Check sheet for the modelled part. Datum: model origin and axes. Units: mm. A direction names the side the tool comes from. Give positions to 0.01 mm unless a question says otherwise; leave off trailing zeros. Write each loop counter-clockwise with the first axis right and the second up, starting at its lowest first coordinate (ties: lowest second). Pieces come first, ordered by that corner, then holes. Notation, with made-up numbers: M -24.5,12.5 L 9.5,12.5 A25 cw 9.5,28.5 Z; hole C 36.5,-31 d2. An arc over 180 degrees is marked long. One line per item, written item: value. Start each with the question number.
from build123d import *

# Parameters (mm, degrees)
CSK_FOR_M3_SFHCS1_AT_2_COUNT = 2
CSK_FOR_M3_SFHCS1_AT_2_PITCH = 17.67766953
CSK_FOR_M3_SFHCS1_AT_3_COUNT = 2
CSK_FOR_M3_SFHCS1_AT_3_PITCH = 25
CSK_FOR_M3_SFHCS1_AT_4_COUNT = 2
CSK_FOR_M3_SFHCS1_AT_4_PITCH = 17.67766953
BOSS_EXTRUDE3_DEPTH          = 10.75
BOSS_EXTRUDE7_DEPTH          = 2
FILLET6_R                    = 5
SKETCH14_R                   = 1.25
CUT_EXTRUDE2_DEPTH           = 13.75
BOSS_EXTRUDE8_DEPTH          = 12.75
SKETCH16_R                   = 1.25
CUT_EXTRUDE3_DEPTH           = 13.75
FILLET8_R                    = 5
SKETCH17_R                   = 1.5
BOSS_EXTRUDE9_DEPTH          = 1.5
SKETCH20_R                   = 11.625
CUT_EXTRUDE4_DEPTH           = 1.5


with BuildPart() as part:
    # Sketch1 → Revolve1 (revolve)
    with BuildSketch(Plane(origin=(0, 0, 0), x_dir=(0, 0, -1), z_dir=(1, 0, 0))):
        Polygon((5.929940933, 28.5), (-0.458333333, 28.5), (-0.458333333, 17.5), (-0.458333333, 7), (6.541666667, 7), (6.541666667, 8.5), (2.541666667, 8.5), (2.541666667, 9), (2.041666667, 9), (2.041666667, 15), (2.041666667, 26.5), (6.791666667, 26.5), (6.791666667, 27.5), (12.291666667, 27.5), (12.291666667, 28.5), align=None)
    revolve(axis=Axis((0, 0, 0), (0, 0, -1)))

    # Sketch3 → CSK for M3 SFHCS1 (revolve, cut)
    with BuildSketch(Plane(origin=(0, 12.5, -2.041666667), x_dir=(0, 1, 0), z_dir=(1, 0, 0))):
        Polygon((0, 0), (0, 2.5), (1.6, 2.5), (1.6, 1.76), (3.36, 0), align=None)
    csk_for_m3_sfhcs1 = revolve(axis=Axis((0, 12.5, -8.391666667), (0, 0, 1)), mode=Mode.SUBTRACT)

    # CSK for M3 SFHCS1 at 2: CSK for M3 SFHCS1 ×2
    with Locations(*[Vector(-0.707106781, -0.707106781, 0) * (i * CSK_FOR_M3_SFHCS1_AT_2_PITCH) for i in range(1, CSK_FOR_M3_SFHCS1_AT_2_COUNT)]):
        add(csk_for_m3_sfhcs1, mode=Mode.SUBTRACT)

    # CSK for M3 SFHCS1 at 3: CSK for M3 SFHCS1 ×2
    with Locations(*[(0, -i * CSK_FOR_M3_SFHCS1_AT_3_PITCH, 0) for i in range(1, CSK_FOR_M3_SFHCS1_AT_3_COUNT)]):
        add(csk_for_m3_sfhcs1, mode=Mode.SUBTRACT)

    # CSK for M3 SFHCS1 at 4: CSK for M3 SFHCS1 ×2
    with Locations(*[Vector(0.707106781, -0.707106781, 0) * (i * CSK_FOR_M3_SFHCS1_AT_4_PITCH) for i in range(1, CSK_FOR_M3_SFHCS1_AT_4_COUNT)]):
        add(csk_for_m3_sfhcs1, mode=Mode.SUBTRACT)

    # Sketch11 → Boss-Extrude3 (add)
    with BuildSketch(Plane.XY.offset(0.458333333)):
        with BuildLine():
            Line((-22.5, 29.5), (-22.5, 17.492855685))
            ThreePointArc((-22.5, 17.492855685), (0, 28.5), (22.5, 17.492855685))
            Line((22.5, 17.492855685), (22.5, 29.5))
            Line((22.5, 29.5), (-22.5, 29.5))
        make_face()
    extrude(amount=-BOSS_EXTRUDE3_DEPTH)

    # Sketch12 → Boss-Extrude7 (add)
    with BuildSketch(Plane(origin=(0, 0, -10.291666667), x_dir=(-1, 0, 0), z_dir=(0, 0, -1))):
        with BuildLine():
            ThreePointArc((-18.04999995, 22.055554897), (-19.216219586, 21.047254092), (-20.326210311, 19.977366553))
            ThreePointArc((-20.326210311, 19.977366553), (-19.921854076, 19.839957524), (-19.503772735, 19.752818562))
            ThreePointArc((-19.503772735, 19.752818562), (-17.580801654, 21.482234642), (-15.505225986, 23.02518098))
            ThreePointArc((-15.505225986, 23.02518098), (-15.50130674, 23.120741552), (-15.5, 23.216373532))
            ThreePointArc((-15.5, 23.216373532), (-15.515704879, 23.547564583), (-15.562678578, 23.875783453))
            ThreePointArc((-15.562678578, 23.875783453), (-16.830963949, 22.999318523), (-18.04999995, 22.055554897))
        make_face()
        with BuildLine():
            ThreePointArc((-19, 26.716373532), (-21.474873734, 25.691247267), (-22.5, 23.216373532))
            ThreePointArc((-22.5, 23.216373532), (-21.906177566, 21.265955127), (-20.326210311, 19.977366553))
            ThreePointArc((-20.326210311, 19.977366553), (-19.216219586, 21.047254092), (-18.04999995, 22.055554897))
            ThreePointArc((-18.04999995, 22.055554897), (-16.830963949, 22.999318523), (-15.562678578, 23.875783453))
            ThreePointArc((-15.562678578, 23.875783453), (-16.77041873, 25.914329677), (-19, 26.716373532))
        make_face()
        with BuildLine():
            ThreePointArc((-17.5, 23.216373532), (-17.644455815, 22.574111933), (-18.04999995, 22.055554897))
            ThreePointArc((-18.04999995, 22.055554897), (-20.355544185, 23.858635132), (-17.5, 23.216373532))
        make_face(mode=Mode.SUBTRACT)
        with BuildLine():
            ThreePointArc((-20.326210311, 19.977366553), (-21.906177566, 21.265955127), (-22.5, 23.216373532))
            Line((-22.5, 23.216373532), (-22.5, 17.492855685))
            ThreePointArc((-22.5, 17.492855685), (-21.449108862, 18.766612082), (-20.326210311, 19.977366553))
        make_face()
        with BuildLine():
            ThreePointArc((18.049999991, 22.055554863), (16.830963971, 22.999318508), (15.562678578, 23.875783453))
            ThreePointArc((15.562678578, 23.875783453), (15.507956483, 23.452238061), (15.505225986, 23.02518098))
            ThreePointArc((15.505225986, 23.02518098), (17.580801654, 21.482234642), (19.503772735, 19.752818562))
            ThreePointArc((19.503772735, 19.752818562), (19.921854076, 19.839957524), (20.326210311, 19.977366553))
            ThreePointArc((20.326210311, 19.977366553), (19.216219606, 21.047254074), (18.049999991, 22.055554863))
        make_face()
        with BuildLine():
            ThreePointArc((22.5, 23.216373532), (21.474873734, 25.691247267), (19, 26.716373532))
            ThreePointArc((19, 26.716373532), (16.77041873, 25.914329677), (15.562678578, 23.875783453))
            ThreePointArc((15.562678578, 23.875783453), (16.830963971, 22.999318508), (18.049999991, 22.055554863))
            ThreePointArc((18.049999991, 22.055554863), (19.216219606, 21.047254074), (20.326210311, 19.977366553))
            ThreePointArc((20.326210311, 19.977366553), (21.906177566, 21.265955127), (22.5, 23.216373532))
        make_face()
        with BuildLine():
            ThreePointArc((20.5, 23.216373532), (19.642261624, 21.860829359), (18.049999991, 22.055554863))
            ThreePointArc((18.049999991, 22.055554863), (18.357738376, 24.571917706), (20.5, 23.216373532))
        make_face(mode=Mode.SUBTRACT)
        with BuildLine():
            ThreePointArc((20.326210311, 19.977366553), (21.449108862, 18.766612082), (22.5, 17.492855685))
            Line((22.5, 17.492855685), (22.5, 23.216373532))
            ThreePointArc((22.5, 23.216373532), (21.906177566, 21.265955127), (20.326210311, 19.977366553))
        make_face()
    extrude(amount=BOSS_EXTRUDE7_DEPTH)

    # Fillet6
    fillet6_edges = [part.edges().sort_by_distance(p)[0] for p in [
        (-15.562678578, 23.875783453, -11.291666667),
        (22.5, 17.492855685, -5.916666667),
        (-22.5, 17.492855685, -5.916666667),
        (15.562678578, 23.875783453, -11.291666667),
    ]]
    fillet(fillet6_edges, radius=FILLET6_R)

    # Sketch14 → Cut-Extrude2 (cut, through all)
    with BuildSketch(Plane(origin=(0, 0, -12.291666667), x_dir=(-1, 0, 0), z_dir=(0, 0, -1))):
        with Locations((-19, 23.216373532)):
            Circle(SKETCH14_R)
        with Locations((19, 23.216373532)):
            Circle(SKETCH14_R)
    extrude(amount=-CUT_EXTRUDE2_DEPTH, mode=Mode.SUBTRACT)

    # Sketch15 → Boss-Extrude8 (add)
    with BuildSketch(Plane.XY.offset(0.458333333)):
        with BuildLine():
            ThreePointArc((17.858431324, -22.210952943), (21.717335169, -24.676706171), (24.713203436, -21.213203436))
            ThreePointArc((24.713203436, -21.213203436), (24.018744674, -19.120612133), (22.210952943, -17.858431324))
            ThreePointArc((22.210952943, -17.858431324), (20.152543264, -20.152543264), (17.858431324, -22.210952943))
        make_face()
        with BuildLine():
            ThreePointArc((-22.210952943, -17.858431324), (-23.68807717, -23.68807717), (-17.858431324, -22.210952943))
            ThreePointArc((-17.858431324, -22.210952943), (-20.152543264, -20.152543264), (-22.210952943, -17.858431324))
        make_face()
    extrude(amount=-BOSS_EXTRUDE8_DEPTH)

    # Sketch16 → Cut-Extrude3 (cut, through all)
    with BuildSketch(Plane(origin=(0, 0, -12.291666667), x_dir=(-1, 0, 0), z_dir=(0, 0, -1))):
        with Locations((-21.213203436, -21.213203436)):
            Circle(SKETCH16_R)
        with Locations((21.213203436, -21.213203436)):
            Circle(SKETCH16_R)
    extrude(amount=-CUT_EXTRUDE3_DEPTH, mode=Mode.SUBTRACT)

    # Fillet8
    fillet8_edges = [part.edges().sort_by_distance(p)[0] for p in [
        (17.858431324, -22.210952943, -5.916666667),
        (22.210952943, -17.858431324, -5.916666667),
        (-22.210952943, -17.858431324, -5.916666667),
        (-17.858431324, -22.210952943, -5.916666667),
    ]]
    fillet(fillet8_edges, radius=FILLET8_R)

    # Sketch17 → Boss-Extrude9 (add)
    with BuildSketch(Plane.XY.offset(0.458333333)):
        with Locations((8.220116331, 8.220116331)):
            Circle(SKETCH17_R)
        with Locations((8.220116331, -8.220116331)):
            Circle(SKETCH17_R)
        with Locations((-8.220116331, -8.220116331)):
            Circle(SKETCH17_R)
        with Locations((-8.220116331, 8.220116331)):
            Circle(SKETCH17_R)
    extrude(amount=BOSS_EXTRUDE9_DEPTH)

    # Sketch20 → Cut-Extrude4 (cut)
    with BuildSketch(Plane.XY.offset(1.958333333)):
        Circle(SKETCH20_R)
    extrude(amount=-CUT_EXTRUDE4_DEPTH, mode=Mode.SUBTRACT)


solid = part.part
1) Cross-section at A-A (y = -12.5). Record the boundary of the cut face in (x, z).
2) Tool access check on faces 4 (the cylindrical face through (-26.846, -5.961, -9.58)), 5 (the flat face through (22.5, 24, -6)), 6 (the cylindrical face through (9.26, -9.3, 1.2)). Record the directions out of +Z, -Z, +X, -X, +Y, -Y that give a thin tool (end or side, any length) a straight path to the whole face; none if there is none.
3) Cross-section at B-B (x = 0). State how many separate pieces and enclosed holes the cut face has, plus the area to 3 significant figures.
4) Gauge pin test, flat ends, axial feed: pin 1 (5 mm diameter, centred on y = 9.5, z = -10, fed in from -X); pin 2 (6 mm diameter, centred on x = -22.5, y = 20, fed in from +Z); pin 3 (4 mm diameter, centred on y = 20.5, z = -3.5, fed in from +X); pin 4 (3.5 mm diameter, centred on x = -19.5, y = 23, fed in from -Z). Record the tip position at first contact, or that the pin passes through.
5) Material ranges on L1, parallel to X at y = 0, z = -4.8; L2, parallel to Y at x = -19, z = -7.75; L3, parallel to X at y = -7.5, z = -5.75, recorded low to high. Write a range as from..to.
6) Draft check along Y on faces 1 (the flat face through (0, 29.5, -5)), 2 (the flat face through (-9, 9, 1.958)), 3 (the flat face through (-3.3, -8, -2.542)). Enter one of: released by +Y, released by -Y, zero draft, split by the parting line, or undercut.
Data:
1. outline: M -25.61,-12.29 L -24.49,-12.29 L -24.49,-6.79 L -23.37,-6.79 L -23.37,-2.04 L -3.36,-2.04 L -1.6,-0.28 L -1.6,0.46 L -25.61,0.46 Z; M 1.6,-0.28 L 3.36,-2.04 L 23.37,-2.04 L 23.37,-6.79 L 24.49,-6.79 L 24.49,-12.29 L 25.61,-12.29 L 25.61,0.46 L 1.6,0.46 Z
2. face 4: -Z
2. face 5: +Z, -Z, +X, +Y
2. face 6: +Z
3. separate pieces: 4
3. enclosed holes: 0
3. area: 140 mm2
4. pin 1: stops at x = -27.63
4. pin 2: stops at z = 0.46
4. pin 3: stops at x = 22.54
4. pin 4: stops at z = -12.29
5. L1: x = -28.5..-26.5, -8.5..-7, 7..8.5, 26.5..28.5
5. L2: y = -24.05..-19.88, 19.88..21.97, 24.47..29.5
5. L3: x = -27.5..-25.42, -4..4, 25.42..27.5
6. face 1: released by +Y
6. face 2: zero draft
6. face 3: undercut
